Verification items for the finished model (mm, model axes). Face numbers are marked on the shaded views. A direction names the side the tool comes from. Round coordinates to 2 decimals unless told otherwise and drop trailing zeros. Order: outer loops, then holes, each group sorted by start corner. A loop starts at its lowest first (then second) coordinate and runs counter-clockwise, first axis right, second up. Notation, with made-up numbers: (69.5, 84) -> (106.5, 84) arc R9 cw to (106.5, 91) -> close; hole circle Ø11 at (65.25, -5.75). An arc over 180 degrees is marked (long way). Return JSON: item names as keys, results as strings. Group by question number.
1) Section check B-B on y = 52.5. Enter the section's corners in (x, z) (3 decimals), plus the area to 3 significant figures.
2) Section check D-D on z = 16. Enter the section's corners in (x, y).
3) Scan lines: L1, parallel to Z at x = -1.5, y = 58.5 (3 decimals); L2, parallel to Y at x = -50, z = 18; L3, parallel to Y at x = -37, z = 11.5. Record each from-to range of solid material in increasing order.
4) Depth check by flat-ended pin: pin 1 (1.5 mm diameter, centred on x = -94.5, z = -7.5, fed in from +Y); pin 2 (2.5 mm diameter, centred on x = -72.5, z = 1, fed in from +Y); pin 3 (12 mm diameter, centred on y = 56.5, z = -23, fed in from -X). Enter the tip coordinate at first touch or a pass-through.
5) Section check A-A on z = 24.5. Enter the section's corners in (x, y) (3 decimals), plus the area to 3 significant figures.
6) Draft check along X on the marked faces 5, 6 and 7. Enter one of: pulls with the +X half, pulls with the -X half, needs draft (parallel to the pull), parting line crosses it, or undercut.
7) Section check C-C on y = 59.5. Enter the section's corners in (x, z) (3 decimals), plus the area to 3 significant figures.
8) Tool access check on the marked faces 1, 2, 3 and 4. Record the directions out of +Z, -Z, +X, -X, +Y, -Y that give a thin tool (end or side, any length) a straight path to the whole face; none if there is none.
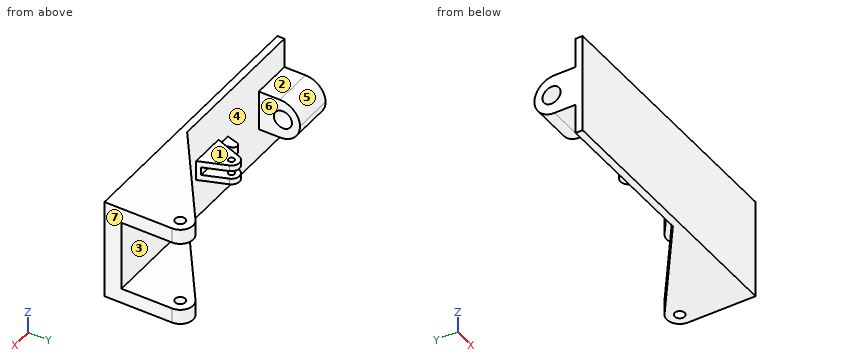
```python
from build123d import *

# Parameters (mm, degrees)
SKETCH1_W           = 171.704
SKETCH1_H           = 4.445
BASE_EXTRUDE_DEPTH  = 31.75
SKETCH4_W           = 25.4
SKETCH4_H           = 30.48
BOSS_EXTRUDE3_DEPTH = 12.7
SKETCH5_R           = 5.715
CUT_EXTRUDE1_DEPTH  = 160.803312245
SKETCH3_R           = 1.905
BOSS_EXTRUDE1_DEPTH = 6.35
SKETCH2_R           = 3.175
BOSS_EXTRUDE2_DEPTH = 31.75
FILLET1_R           = 12.7
CUT_EXTRUDE2_DEPTH  = 2.54
CUT_EXTRUDE4_DEPTH  = 22.225
BOSS_EXTRUDE4_DEPTH = 2.54


with BuildPart() as part:
    # Sketch1 → Base-Extrude (new, symmetric)
    with BuildSketch(Plane.XY):
        with Locations((-59.590145552, 27.636826085)):
            Rectangle(SKETCH1_W, SKETCH1_H)
    extrude(amount=BASE_EXTRUDE_DEPTH, both=True)

    # Sketch4 → Boss-Extrude3 (add, symmetric)
    with BuildSketch(Plane.XY):
        with Locations((-132.742145552, 40.654326085)):
            Rectangle(SKETCH4_W, SKETCH4_H)
    extrude(amount=BOSS_EXTRUDE3_DEPTH, both=True)

    # Sketch5 → Cut-Extrude1 (cut, through all)
    with BuildSketch(Plane(origin=(-120.042145552, 0, 0), x_dir=(0, 0, -1), z_dir=(1, 0, 0))):
        with Locations((0, 45.096262506)):
            Circle(SKETCH5_R)
    extrude(amount=-CUT_EXTRUDE1_DEPTH, mode=Mode.SUBTRACT)

    # Sketch3 → Boss-Extrude1 (add, symmetric)
    with BuildSketch(Plane.XY):
        with BuildLine():
            Line((-81.627185552, 25.414326085), (-56.227185552, 25.414326085))
            Line((-56.227185552, 25.414326085), (-64.162927469, 46.859284036))
            ThreePointArc((-64.162927469, 46.859284036), (-68.927185552, 50.176262506), (-73.691443636, 46.859284036))
            Line((-73.691443636, 46.859284036), (-81.627185552, 25.414326085))
        make_face()
        with Locations((-68.927185552, 45.096262506)):
            Circle(SKETCH3_R, mode=Mode.SUBTRACT)
    extrude(amount=BOSS_EXTRUDE1_DEPTH, both=True)

    # Sketch2 → Boss-Extrude2 (add, symmetric)
    with BuildSketch(Plane.XY):
        with BuildLine():
            Line((-55.018145552, 25.414326085), (26.261854448, 25.414326085))
            Line((26.261854448, 25.414326085), (26.261854448, 68.187926085))
            ThreePointArc((26.261854448, 68.187926085), (21.835266898, 75.424218635), (13.377029184, 74.77860112))
            Line((13.377029184, 74.77860112), (-55.018145552, 25.414326085))
        make_face()
        with Locations((18.133854448, 68.187926085)):
            Circle(SKETCH2_R, mode=Mode.SUBTRACT)
    extrude(amount=BOSS_EXTRUDE2_DEPTH, both=True)

    # Fillet1
    fillet1_edges = [part.edges().sort_by_distance(p)[0] for p in [
        (-132.742145552, 55.894326085, 12.7),
        (-132.742145552, 55.894326085, -12.7),
    ]]
    fillet(fillet1_edges, radius=FILLET1_R - 0.0001)  # a hair under: the kernel refuses the full size

    # Sketch6 → Cut-Extrude2 (cut, symmetric)
    with BuildSketch(Plane.XY):
        with BuildLine():
            Line((-79.042374828, 32.399326085), (-58.811996277, 32.399326085))
            Line((-58.811996277, 32.399326085), (-64.162927469, 46.859284036))
            ThreePointArc((-64.162927469, 46.859284036), (-68.927185552, 50.176262506), (-73.691443636, 46.859284036))
            Line((-73.691443636, 46.859284036), (-79.042374828, 32.399326085))
        make_face()
    extrude(amount=CUT_EXTRUDE2_DEPTH, both=True, mode=Mode.SUBTRACT)

    # Sketch7 → Cut-Extrude4 (cut, symmetric)
    with BuildSketch(Plane.XY):
        with BuildLine():
            Line((13.377029184, 74.77860112), (-40.061460566, 36.209326085))
            Line((-40.061460566, 36.209326085), (26.261854448, 36.209326085))
            Line((26.261854448, 36.209326085), (26.261854448, 68.187926085))
            ThreePointArc((26.261854448, 68.187926085), (21.835266898, 75.424218635), (13.377029184, 74.77860112))
        make_face()
    extrude(amount=CUT_EXTRUDE4_DEPTH, both=True, mode=Mode.SUBTRACT)

    # Sketch8 → Boss-Extrude4 (add, symmetric)
    with BuildSketch(Plane.XY):
        with BuildLine():
            Line((-90.484109136, 25.414326085), (-79.221861969, 25.414326085))
            Line((-79.221861969, 25.414326085), (-82.40622809, 36.840418981))
            ThreePointArc((-82.40622809, 36.840418981), (-84.852985552, 38.698526085), (-87.299743015, 36.840418981))
            Line((-87.299743015, 36.840418981), (-90.484109136, 25.414326085))
        make_face()
    extrude(amount=BOSS_EXTRUDE4_DEPTH, both=True)


solid = part.part
```
Check result:
{
 "1": {"outline": "(-145.442, -8.643) -> (-120.042, -8.643) -> (-120.042, 8.643) -> (-145.442, 8.643) -> close; (-17.49, -31.75) -> (26.262, -31.75) -> (26.262, -22.225) -> (-17.49, -22.225) -> close; (-17.49, 22.225) -> (26.262, 22.225) -> (26.262, 31.75) -> (-17.49, 31.75) -> close", "area": "1,270 mm^2"},
 "2": {"outline": "(-145.44, 25.41) -> (26.26, 25.41) -> (26.26, 36.21) -> (-40.06, 36.21) -> (-48.86, 29.86) -> (-145.44, 29.86) -> close"},
 "3": {"L1": "-31.75 to -22.225, 22.225 to 31.75", "L2": "25.41 to 29.86", "L3": "25.41 to 36.21"},
 "4": {"pin 1": "y = 29.86", "pin 2": "y = 32.4", "pin 3": "x = -20.26"},
 "5": {"outline": "(-145.442, 25.414) -> (26.262, 25.414) -> (26.262, 68.188) arc R8.128 ccw to (13.377, 74.779) -> (-48.86, 29.859) -> (-145.442, 29.859) -> close; hole circle Ø6.35 at (18.134, 68.188)", "area": "2,710 mm^2"},
 "6": {"face 5": "needs draft", "face 6": "undercut", "face 7": "pulls with the +X half"},
 "7": {"outline": "(-7.792, -31.75) -> (26.262, -31.75) -> (26.262, -22.225) -> (-7.792, -22.225) -> close; (-7.792, 22.225) -> (26.262, 22.225) -> (26.262, 31.75) -> (-7.792, 31.75) -> close", "area": "649 mm^2"},
 "8": {"face 1": "+Z, +Y", "face 2": "+Z, -X, +Y", "face 3": "+X, +Y", "face 4": "+Y"}
}
